Geometry: final body of the model. Coordinates: model frame, mm. Give positions to 0.01 mm unless a question says otherwise; leave off trailing zeros. Order: outer loops, then holes, each group sorted by start corner. A loop starts at its lowest first (then second) coordinate and runs counter-clockwise, first axis right, second up. Notation, with made-up numbers: (-34, 4.5) -> (22, 4.5) arc R16 ccw to (22, 24.5) -> close; hole circle Ø7 at (80, -21). An arc over 180 degrees is marked (long way). Write item = value, one per line.
```python
from build123d import *

# Parameters (mm, degrees)
F1_DEPTH = 10
F4_D     = 5
F4_DEPTH = 5
F4_TIP   = 1.5021515476


with BuildPart() as f1:
    # F0 (on Front) → F1 (new body)
    with BuildSketch(Plane.XZ):
        with BuildLine():
            Line((-10, 0), (0, 0))
            Line((0, 0), (0, 10))
            ThreePointArc((0, 10), (-5, 5), (-10, 10))
            Line((-10, 10), (-10, 0))
        make_face()
        with BuildLine():
            Line((-10, 10), (0, 10))
            ThreePointArc((0, 10), (-5, 15), (-10, 10))
        make_face()
        with BuildLine():
            ThreePointArc((-10, 10), (-5, 5), (0, 10))
            Line((0, 10), (-10, 10))
        make_face()
    extrude(amount=F1_DEPTH)

    # F4
    with Locations(Plane(origin=(0, 0, 0), x_dir=(1, 0, 0), z_dir=(0, 0, -1))):
        with Locations((-5.0305076875, 4.9831778742)):
            Hole(F4_D / 2, depth=F4_DEPTH)
            with Locations((0, 0, -(F4_DEPTH + F4_TIP / 2))):  # 118° drill point
                Cone(0, F4_D / 2, F4_TIP, mode=Mode.SUBTRACT)


solid = f1.part
```
1) Section query D-D (x = -8.5). Output: boundary loops of the cut face in (y, z).
Check sheet entries:
outline = (-10, 0) -> (0, 0) -> (0, 13.57) -> (-10, 13.57) -> close
2) Line query: line 1 (X direction, y = -4, z = 3); line 2 (X direction, y = -3.25, z = 12.25); line 3 (X direction, y = -7.5, z = 14). Output: solid intervals per line, ascending. Write a range as from..to.
Check sheet entries:
line_1 = -10..-7.33, -2.73..0
line_2 = -9.47..-0.53
line_3 = -8..-2
3) First-contact query: P1, Ø4, axis at x = -5.03, y = -4.98, coming from the -Z side; P2, Ø3, axis at x = -6, y = -7.5, coming from the +Z side; P3, Ø1, axis at x = -6.5, y = -7, coming from the +Z side. Flat tips, straight axial feed; report the tip coordinate or a pass-through.
Check sheet entries:
P1 = 5.3
P2 = 15
P3 = 14.9
4) Section query B-B (x = -0.25). Output: boundary loops of the cut face in (y, z), plus the area to 3 significant figures.
Check sheet entries:
outline = (-10, 0) -> (0, 0) -> (0, 11.56) -> (-10, 11.56) -> close
area = 116 mm²
5) Section query A-A (z = 5.75). Output: boundary loops of the cut face in (x, y), plus the area to 3 significant figures.
Check sheet entries:
outline = (-10, -10) -> (0, -10) -> (0, 0) -> (-10, 0) -> close; hole circle Ø2.5 at (-5.03, -4.98)
area = 95.1 mm²
6) Section query C-C (z = 2). Output: boundary loops of the cut face in (x, y).
Check sheet entries:
outline = (-10, -10) -> (0, -10) -> (0, 0) -> (-10, 0) -> close; hole circle Ø5 at (-5.03, -4.98)
7) Mould query, pull axis Y, two halves, no side actions, for faces 1 (the face through (-4.63, -4.82, 6.24)), 2 (the face through (-7.415, -5.734, 2.535)), 3 (the face through (-5, -10, 8)), 4 (the face through (-5, 0, 8)). Classes: +Y half, -Y half, draft (parallel to the pull), parting line (faces both ways), or undercut.
Check sheet entries:
face_1 = undercut
face_2 = undercut
face_3 = -Y half
face_4 = +Y half
